Design review of the part shown in the three views and the two pictorial views. Dimensions are in mm from the part's minimum x, y and z. A direction names the side the tool comes from. Round coordinates to 2 decimals unless told otherwise and drop trailing zeros. Loops run counter-clockwise (first coordinate to the right, second up) from the corner with the lowest first, then second, coordinate; pieces in that order, holes last. Notation, with made-up numbers: (76.25, 39) -> (90.25, 39) arc R28 cw to (90.25, 67) -> close; hole circle Ø7 at (41.5, 30). An arc over 180 degrees is marked (long way). One line per question, with ' | ' between items. Start each with the question number.
1. Wall thickness on line 1 along X through (y, z) = (8, 13); line 2 along Y through (x, z) = (5, 9); line 3 along X through (y, z) = (4.75, 6.75): over which ranges is each line inside the solid? List them lowest first.
2. Consider section B-B (y = 13.75). Write out the cut boundary in (x, z), and give its area (3 significant figures).
3. Draft analysis for pull direction X (two halves, no side actions). For the marked faces 3, 4, 5 and 6, state which applies: pulls with the +X half, pulls with the -X half, needs draft (parallel to the pull), parting line crosses it, or undercut.
4. Consider section A-A (z = 10). Count the separate pieces of the cut face and the enclosed holes in it, and give its area (3 significant figures).
5. Consider section D-D (x = 19). Write out the cut boundary in (y, z).
6. For pin 1 Ø4 at (x, z) = (42.5, 10) entering from -Y; pin 2 Ø3.5 at (x, z) = (19, 4) entering from +Y; pin 3 Ø4 at (x, z) = (53.5, 4.5) entering from -Y, all flat-tipped, find the tip position at first contact; note any pin that passes through.
7. For the marked faces 1 and 2, list the 3-axis set-ups (+Z, -Z, +X, -X, +Y, -Y) from which the entire face can be reached by the end or side of a thin tool; tool diameter is ignored.
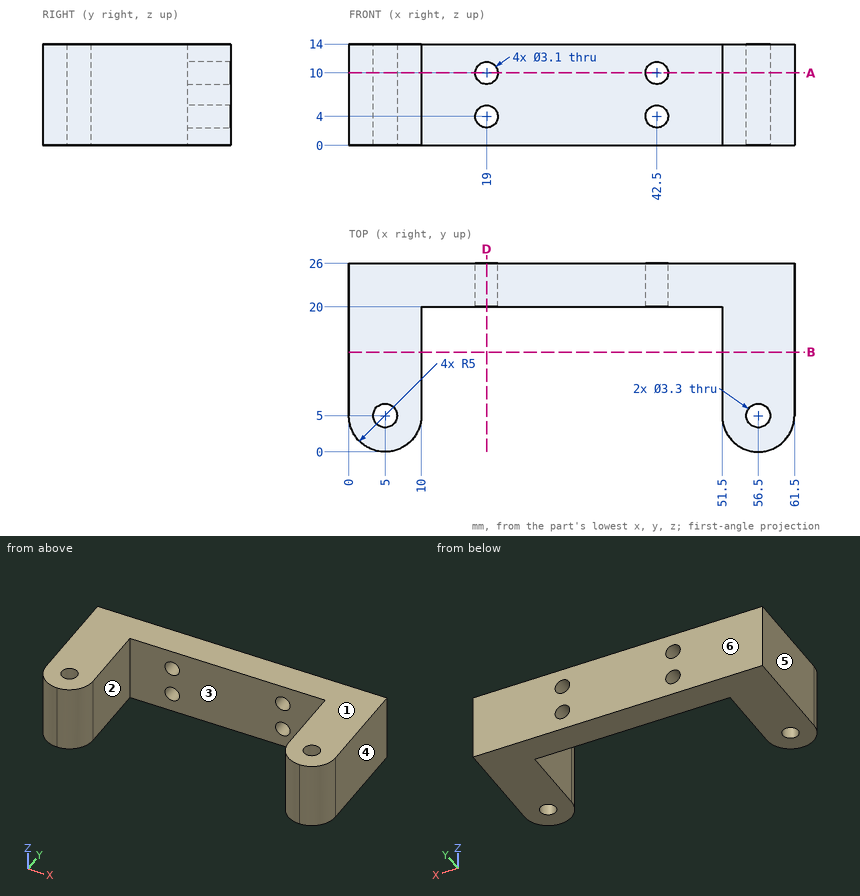
Answer block:
1) line 1: x = 0 to 10, 51.5 to 61.5 | line 2: y = 0 to 3.35, 6.65 to 26 | line 3: x = 0.01 to 3.37, 6.63 to 9.99, 51.51 to 54.87, 58.13 to 61.49
2) outline: (0, 0) -> (10, 0) -> (10, 14) -> (0, 14) -> close; (51.5, 0) -> (61.5, 0) -> (61.5, 14) -> (51.5, 14) -> close | area: 280 mm2
3) face 3: undercut | face 4: pulls with the +X half | face 5: pulls with the -X half | face 6: needs draft
4) separate pieces: 3 | enclosed holes: 2 | area: 693 mm2
5) outline: (20, 0) -> (26, 0) -> (26, 2.45) -> (20, 2.45) -> close; (20, 5.55) -> (26, 5.55) -> (26, 8.45) -> (20, 8.45) -> close; (20, 11.55) -> (26, 11.55) -> (26, 14) -> (20, 14) -> close
6) pin 1: stops at y = 20 | pin 2: stops at y = 26 | pin 3: stops at y = 0.1
7) face 1: +Z, +X, -X, +Y, -Y | face 2: +Z, -Z, -Y
